from build123d import *

# Parameters (mm, degrees)
SKETCH1_W                  = 24
SKETCH1_H                  = 43
PCB_DEPTH                  = 1.25
SKETCH2_W                  = 22
SKETCH2_H                  = 34
RF_CASING_DEPTH            = 3
SKETCH3_W                  = 6.5
SKETCH3_H                  = 6.5
RF_CONNECTOR_BACK_DEPTH    = 1.5
SKETCH4_R                  = 3
RF_CONNECTOR_THREADS_DEPTH = 11
SKETCH5_W                  = 6.5
SKETCH5_H                  = 3
RF_CONNECTOR_PINS_DEPTH    = 4


with BuildPart() as part:
    # Sketch1 → PCB (new body)
    with BuildSketch(Plane(origin=(0, 0, 0), x_dir=(1, 0, 0), z_dir=(0, 1, 0))):
        Rectangle(SKETCH1_W, SKETCH1_H)
    extrude(amount=PCB_DEPTH)

    # Sketch2 → RF Casing (add)
    with BuildSketch(Plane(origin=(0, 1.25, 0), x_dir=(1, 0, 0), z_dir=(0, 1, 0))):
        with Locations((0, 1.5)):
            Rectangle(SKETCH2_W, SKETCH2_H)
    extrude(amount=RF_CASING_DEPTH)

    # Sketch3 → RF Connector Back (add)
    with BuildSketch(Plane.XY.offset(21.5)):
        with Locations((-6.75, 2)):
            Rectangle(SKETCH3_W, SKETCH3_H)
    extrude(amount=RF_CONNECTOR_BACK_DEPTH)

    # Sketch4 → RF Connector Threads (add)
    with BuildSketch(Plane.XY.offset(23)):
        with Locations((-6.75, 2)):
            Circle(SKETCH4_R)
    extrude(amount=RF_CONNECTOR_THREADS_DEPTH)

    # Sketch5 → RF Connector Pins (add)
    with BuildSketch(Plane(origin=(0, 0, 21.5), x_dir=(-1, 0, 0), z_dir=(0, 0, -1))):
        with Locations((6.75, 0.625)):
            Rectangle(SKETCH5_W, SKETCH5_H)
    extrude(amount=RF_CONNECTOR_PINS_DEPTH)


solid = part.part
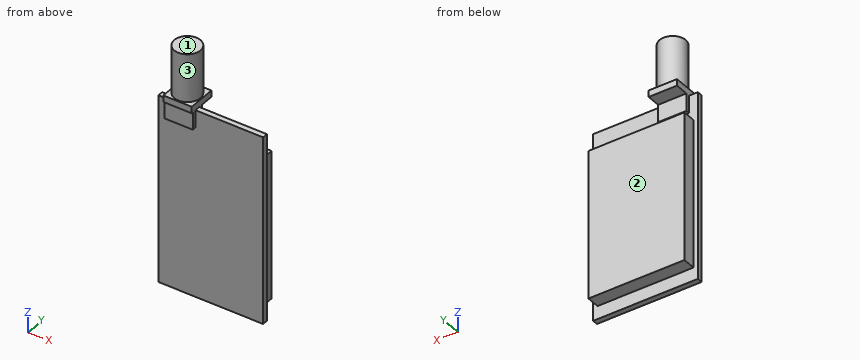
Work out the finished part from the listing and answer in its coordinate system (mm). Face numbers are marked on the shaded views. A direction names the side the tool comes from. Give positions to 0.01 mm unless a question says otherwise; leave off trailing zeros. Order: outer loops, then holes, each group sorted by start corner. A loop starts at its lowest first (then second) coordinate and runs counter-clockwise, first axis right, second up. Notation, with made-up numbers: (48.25, 86) -> (70.25, 86) arc R25 ccw to (70.25, 100) -> close; hole circle Ø2 at (70.25, 72). An arc over 180 degrees is marked (long way). One line per item, written item: value.
Item 1: Find section C-C, the plane y = 3.75. Give the vertices of the cut face in (x, z).
Answer sheet:
outline: (-11, -18.5) -> (11, -18.5) -> (11, 15.5) -> (-11, 15.5) -> close; (-10, 21.5) -> (-3.5, 21.5) -> (-3.5, 23) -> (-4.31, 23) -> (-4.31, 34) -> (-9.19, 34) -> (-9.19, 23) -> (-10, 23) -> close
Item 2: Find section A-A, the plane x = 3.75. Give the vertices of the cut face in (y, z).
Answer sheet:
outline: (0, -21.5) -> (1.25, -21.5) -> (1.25, -18.5) -> (4.25, -18.5) -> (4.25, 15.5) -> (1.25, 15.5) -> (1.25, 21.5) -> (0, 21.5) -> close
Item 3: Find section D-D, the plane y = 0.5. Give the vertices of the cut face in (x, z).
Answer sheet:
outline: (-12, -21.5) -> (12, -21.5) -> (12, 21.5) -> (-3.5, 21.5) -> (-3.5, 23) -> (-4.15, 23) -> (-4.15, 34) -> (-9.35, 34) -> (-9.35, 23) -> (-10, 23) -> (-10, 21.5) -> (-12, 21.5) -> close
Item 4: A tool of negligible diameter and unlimited length cuts with its end or side. For the marked faces 1, 2 and 3, from which of +Z, -Z, +X, -X, +Y, -Y can it reach the whole face along a straight path? Write none if from no direction.
Answer sheet:
face 1: +Z, +X, -X, +Y, -Y
face 2: -Z, +X, -X, +Y
face 3: +Z
Item 5: Find section B-B, the plane z = 2. Give the vertices of the cut face in (x, y).
Answer sheet:
outline: (-12, 0) -> (12, 0) -> (12, 1.25) -> (11, 1.25) -> (11, 4.25) -> (-11, 4.25) -> (-11, 1.25) -> (-12, 1.25) -> close
Item 6: Straight lines are drawn through the part: probe 1 along Y at (x, z) = (-5.25, -13.5); probe 2 along Z at (x, y) = (0.25, 2.5); probe 3 along X at (y, z) = (3.75, 2). For each, find the intervals that lie inside material, in ascending order.
Answer sheet:
probe 1: 0 to 4.25
probe 2: -18.5 to 15.5
probe 3: -11 to 11
Item 7: Flat-ended cylindrical pins translate along their axes: P1, Ø3, axis at x = 2, z = -2.5, coming from the -Y side; P2, Ø0.9, axis at x = -8, y = 3.5, coming from the -Z side; P3, Ø1, axis at x = 0.5, y = 0.5, coming from the +Z side. Find the tip coordinate at first contact, or state that the pin passes through.
Answer sheet:
P1: y = 0
P2: z = -18.5
P3: z = 21.5
